For this review, take the finished solid that the model builds, in its own axes (mm). Coordinates: 2 decimals unless noted, no trailing zeros. Order: outer loops, then holes, each group sorted by start corner. A loop starts at its lowest first (then second) coordinate and runs counter-clockwise, first axis right, second up. Notation, with made-up numbers: (6.25, 85) -> (59.25, 85) arc R6 cw to (59.25, 93) -> close; hole circle Ø10 at (31, -13). An arc over 180 degrees is marked (long way). Answer as a JSON object with one key per item and string values. Group by question number.
1) Add section C-C, the plane z = 1.3. Write out the cut boundary in (x, y).
2) Wall thickness on L1, parallel to Y at x = 6, z = 1.5; L2, parallel to X at y = -11, z = 0.7; L3, parallel to X at y = -3.5, z = 0.45: over which ranges is each line inside the solid? List them lowest first.
3) Add section A-A, the plane x = 7.5. Write out the cut boundary in (y, z).
4) Add section B-B, the plane y = -12.5. Write out the cut boundary in (x, z), then the cut area to 3 significant figures.
5) Add section D-D, the plane y = -22.5. Write out the cut boundary in (x, z), then the cut area to 3 significant figures.
Autodesk Inventor part; units mm, degrees
ref_plane "YZ Plane" through (0, 0, 0) normal (1, 0, 0) x (0, 1, 0)
ref_plane "XZ Plane" through (0, 0, 0) normal (0, 1, 0) x (-1, 0, 0)
ref_plane "XY Plane" through (0, 0, 0) normal (0, 0, 1) x (1, 0, 0)
sketch "Sketch1" plane through (0, 0, 0) normal (0, 0, 1) x (1, 0, 0)
  line L0 (0, 0) -> (0, -25)
  line L1 (0, -25) -> (70, -25)
  line L2 (70, -25) -> (70, 0)
  line L3 (70, 0) -> (0, 0)
  dimension "d0" = 25
  dimension "d1" = 70
extrude "Extrusion1" add sketch "Sketch1" along normal blind 3
fillet "Fillet1" radius 5 1 edges at (70, 0, 1.5)
fillet "Fillet2" radius 5 1 edges at (70, -25, 1.5)
fillet "Fillet3" radius 5 1 edges at (0, -25, 1.5)
fillet "Fillet4" radius 5 1 edges at (0, 0, 1.5)
sketch "Sketch2" plane through (0, 0, 0) normal (0, 0, -1) x (-1, 0, 0)
  circle A0 centre (-62.4991, -12.5) radius 2.5
  circle A1 centre (-7.5, -12.5) radius 2.5
  point P0 (0, 0)
extrude "Extrusion2" cut sketch "Sketch2" against normal through all
properties part number "new connect acr" material "Glass"
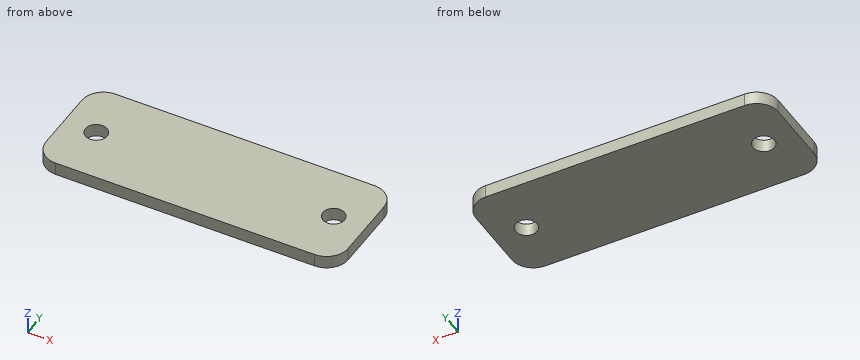
Output values:
{
 "1": {"outline": "(0, -20) arc R5 ccw to (5, -25) -> (65, -25) arc R5 ccw to (70, -20) -> (70, -5) arc R5 ccw to (65, 0) -> (5, 0) arc R5 ccw to (0, -5) -> close; hole circle Ø5 at (7.5, -12.5); hole circle Ø5 at (62.5, -12.5)"},
 "2": {"L1": "y = -25 to -14.5, -10.5 to 0", "L2": "x = 0 to 5.5, 9.5 to 60.5, 64.5 to 70", "L3": "x = 0.23 to 69.77"},
 "3": {"outline": "(-25, 0) -> (-15, 0) -> (-15, 3) -> (-25, 3) -> close; (-10, 0) -> (0, 0) -> (0, 3) -> (-10, 3) -> close"},
 "4": {"outline": "(0, 0) -> (5, 0) -> (5, 3) -> (0, 3) -> close; (10, 0) -> (60, 0) -> (60, 3) -> (10, 3) -> close; (65, 0) -> (70, 0) -> (70, 3) -> (65, 3) -> close", "area": "180 mm²"},
 "5": {"outline": "(0.67, 0) -> (69.33, 0) -> (69.33, 3) -> (0.67, 3) -> close", "area": "206 mm²"}
}
